from build123d import *

# Parameters (mm, degrees)
F0_R     = 1.1
F1_DEPTH = 2
F3_DEPTH = 1.2
F4_R     = 1


with BuildPart() as f1:
    # F0 (on Right) → F1 (new body)
    with BuildSketch(Plane.YZ):
        with BuildLine():
            Line((-4.5, 0), (10.5, 0))
            Line((10.5, 0), (2.638459, 14.527772))
            ThreePointArc((2.638459, 14.527772), (-0.571654, 16.045032), (-2.981013, 13.436989))
            Line((-2.981013, 13.436989), (-4.5, 0))
        make_face()
        with Locations((0, 13.1)):
            Circle(F0_R, mode=Mode.SUBTRACT)
    extrude(amount=F1_DEPTH)

    # F2 (on face) → F3 (cut)
    with BuildSketch(Plane(origin=(0, 0, 0), x_dir=(0, -1, 0), z_dir=(-1, 0, 0))):
        Polygon((-3.112502, 10.5), (-7.982751, 1.5), (2.820878, 1.5), (1.803471, 10.5), align=None)
    extrude(amount=-F3_DEPTH, mode=Mode.SUBTRACT)

    # F4
    f4_edges = [f1.edges().sort_by_distance(p)[0] for p in [
        (0.6, 3.112502, 10.5),
        (0.6, -1.803471, 10.5),
        (0.6, -2.820878, 1.5),
        (0.6, 7.982751, 1.5),
        (1.2, 5.547626, 6),
        (1.2, 2.580936, 1.5),
        (1.2, -2.312175, 6),
        (1.2, 0.654515, 10.5),
    ]]
    fillet(f4_edges, radius=F4_R)


solid = f1.part
Read the model definition and answer for the solid it produces. Units are mm, in the model's axes. A direction names the side the tool comes from. Round coordinates to 2 decimals unless told otherwise and drop trailing zeros. Loops run counter-clockwise (first coordinate to the right, second up) from the corner with the lowest first, then second, coordinate; pieces in that order, holes last. Notation, with made-up numbers: (-3, 42) - (21, 42) arc R26 cw to (21, 81) - close; hole circle Ø4 at (-1, 7.5). An arc over 180 degrees is marked (long way). One line per question, with ' | ' between items. Start each with the question number.
Q1. For faces 1 (the flat face through (0.986, 6.624, 7.162)), 2 (the flat face through (1.2, 1, 5)), determine the directions among +Z, -Z, +X, -X, +Y, -Y from which every point of the face is accessible in a straight line to the end or side of a thin tool.
Q2. Section D-D on z = 14.75 is taken. Give the vertices of the cut face in (x, y), plus the area to 3 significant figures.
Q3. Flat-ended cylindrical pins translate along their axes: pin 1 (1.3 mm diameter, centred on y = 0, z = 13.1, fed in from -X); pin 2 (5.5 mm diameter, centred on y = 2.5, z = 5.5, fed in from -X). Find the tip coordinate at first contact, or state that the pin passes through.
Q4. Section A-A on y = 0 is taken. Give the vertices of the cut face in (x, z), plus the area to 3 significant figures.
Q5. Section B-B on z = 12.75 is taken. Give the vertices of the cut face in (x, y).
Q6. For a pull along Y with two mould halves and no side action, classify faces 3 (the flat face through (0.99, -3.73, 6.81)), 4 (the cylindrical face through (0.9, -2.01, 6.13)), 5 (the flat face through (0, 4, 10)) as +Y half, -Y half, draft (parallel to the pull), parting line (faces both ways), or undercut.
Q7. Section C-C on x = 0.65 is taken. Give the vertices of the cut face in (y, z).
Q8. Find the intervals of material crossed by L1, parallel to Z at x = 0.9, y = 0; L2, parallel to Z at x = 0.7, y = 0; L3, parallel to X at y = 2.5, z = 9, in increasing order.
Established:
1) face 1: +Z, +X, -X, +Y | face 2: -X
2) outline: (0, -2.51) - (2, -2.51) - (2, 2.51) - (0, 2.51) - close | area: 10.0 mm²
3) pin 1: through | pin 2: x = 0.76
4) outline: (0, 0) - (2, 0) - (2, 12) - (0, 12) - (0, 10.5) - (0.2, 10.5) arc R1 cw to (1.2, 9.5) - (1.2, 2.5) arc R1 cw to (0.2, 1.5) - (0, 1.5) - close; (0, 14.2) - (2, 14.2) - (2, 16.1) - (0, 16.1) - close | area: 17.4 mm²
5) outline: (0, -3.06) - (2, -3.06) - (2, -1.04) - (0, -1.04) - close; (0, 1.04) - (2, 1.04) - (2, 3.6) - (0, 3.6) - close
6) face 3: -Y half | face 4: undercut | face 5: draft
7) outline: (-4.5, 0) - (10.5, 0) - (2.64, 14.53) arc R3 ccw to (-2.98, 13.44) - close; hole (-2.59, 2.6) arc R0.89 ccw to (-1.7, 1.61) - (6.3, 1.61) arc R0.89 ccw to (7.09, 2.93) - (3.3, 9.93) arc R0.89 ccw to (2.52, 10.39) - (-0.91, 10.39) arc R0.89 ccw to (-1.8, 9.6) - close; hole circle Ø2.2 at (0, 13.1)
8) L1: 0 to 1.79, 10.21 to 12, 14.2 to 16.1 | L2: 0 to 1.63, 10.37 to 12, 14.2 to 16.1 | L3: 1.2 to 2
